Here's how the part is built. I have some questions about the finished solid (model axes, mm). Round coordinates to 2 decimals unless told otherwise and drop trailing zeros. Loops run counter-clockwise (first coordinate to the right, second up) from the corner with the lowest first, then second, coordinate; pieces in that order, holes last. Notation, with made-up numbers: (3.25, 41.25) - (37.25, 41.25) arc R29 cw to (37.25, 75.25) - close; hole circle Ø1 at (-29, -30.5). An arc over 180 degrees is marked (long way). Return JSON: item names as keys, results as strings. Group by question number.
```python
from build123d import *

# Parameters (mm, degrees)
SKETCH2_W                                     = 2006.6
SKETCH2_H                                     = 762
BOSS_EXTRUDE1_DEPTH                           = 25.4
BOSS_EXTRUDE4_DEPTH                           = 25.4
F_1_4_20_TAPPED_HOLE1_D                       = 5.1054
SKETCH5_R                                     = 215.9
CUT_EXTRUDE2_DEPTH                            = 26.4
SKETCH10_W                                    = 304.8
SKETCH10_H                                    = 762
CUT_EXTRUDE5_DEPTH                            = 26.4
SKETCH31_W                                    = 381
SKETCH31_H                                    = 82.55
CUT_EXTRUDE8_DEPTH                            = 26.4
CUT_EXTRUDE9_DEPTH                            = 26.4
CUT_EXTRUDE10_DEPTH                           = 26.4
SKETCH41_W                                    = 838.2
SKETCH41_H                                    = 457.2
CUT_EXTRUDE11_DEPTH                           = 26.4
CBORE_FOR_1_4_SOCKET_HEAD_CAP_SCREW1_AT_COUNT = 2
CBORE_FOR_1_4_SOCKET_HEAD_CAP_SCREW1_AT_PITCH = 204.781346807
CBORE_FOR_1_4_SOCKET_HEAD_CAP_SCREW1_2_COUNT  = 2
CBORE_FOR_1_4_SOCKET_HEAD_CAP_SCREW1_2_PITCH  = 618.530419624
CBORE_FOR_1_4_SOCKET_HEAD_CAP_SCREW1_3_COUNT  = 2
CBORE_FOR_1_4_SOCKET_HEAD_CAP_SCREW1_3_PITCH  = 819.912629492
CBORE_FOR_1_4_SOCKET_HEAD_CAP_SCREW1_4_COUNT  = 2
CBORE_FOR_1_4_SOCKET_HEAD_CAP_SCREW1_4_PITCH  = 813.196778154


with BuildPart() as part:
    # Sketch2 → Boss-Extrude1 (new body)
    with BuildSketch(Plane(origin=(0, 0, 0), x_dir=(1, 0, 0), z_dir=(0, 1, 0))):
        with Locations((596.720248579, 143.454782609)):
            Rectangle(SKETCH2_W, SKETCH2_H)
    extrude(amount=BOSS_EXTRUDE1_DEPTH)

    # Sketch63 → Boss-Extrude4 (add)
    with BuildSketch(Plane(origin=(0, 25.4, 0), x_dir=(1, 0, 0), z_dir=(0, 1, 0))):
        with BuildLine():
            Line((368.120248579, -237.545217391), (763.550813985, -237.545217391))
            Line((763.550813985, -237.545217391), (761.820248579, -275.645217391))
            Line((761.820248579, -275.645217391), (364.731895319, -275.645217391))
            ThreePointArc((364.731895319, -275.645217391), (367.271491927, -256.670403258), (368.120248579, -237.545217391))
        make_face()
    extrude(amount=-BOSS_EXTRUDE4_DEPTH)

    # 1/4-20 Tapped Hole1 (through all)
    with Locations(Plane(origin=(0, 25.4, 0), x_dir=(1, 0, 0), z_dir=(0, 1, 0))):
        with Locations((736.420248579, -262.945217391)):
            Hole(F_1_4_20_TAPPED_HOLE1_D / 2)

    # Sketch5 → Cut-Extrude2 (cut, through all)
    with BuildSketch(Plane(origin=(0, 25.4, 0), x_dir=(1, 0, 0), z_dir=(0, 1, 0))):
        with Locations((152.220248579, -237.545217391)):
            Circle(SKETCH5_R)
    extrude(amount=-CUT_EXTRUDE2_DEPTH, mode=Mode.SUBTRACT)

    # Sketch10 → Cut-Extrude5 (cut, through all)
    with BuildSketch(Plane(origin=(0, 25.4, 0), x_dir=(1, 0, 0), z_dir=(0, 1, 0))):
        with Locations((-254.179751421, 143.454782609)):
            Rectangle(SKETCH10_W, SKETCH10_H)
    extrude(amount=-CUT_EXTRUDE5_DEPTH, mode=Mode.SUBTRACT)

    # Sketch31 → Cut-Extrude8 (cut, through all)
    with BuildSketch(Plane(origin=(0, 25.4, 0), x_dir=(1, 0, 0), z_dir=(0, 1, 0))):
        with Locations((-216.079751421, -196.270217391)):
            Rectangle(SKETCH31_W, SKETCH31_H)
    extrude(amount=-CUT_EXTRUDE8_DEPTH, mode=Mode.SUBTRACT)

    # Sketch39 → Cut-Extrude9 (cut, through all)
    with BuildSketch(Plane(origin=(0, 25.4, 0), x_dir=(1, 0, 0), z_dir=(0, 1, 0))):
        with BuildLine():
            Line((-101.779751421, 480.875272294), (-101.779751421, 524.454782609))
            Line((-101.779751421, 524.454782609), (152.220248579, 524.454782609))
            ThreePointArc((152.220248579, 524.454782609), (23.36454079, 513.480885065), (-101.779751421, 480.875272294))
        make_face()
    extrude(amount=-CUT_EXTRUDE9_DEPTH, mode=Mode.SUBTRACT)

    # Sketch40 → Cut-Extrude10 (cut, through all)
    with BuildSketch(Plane(origin=(0, 25.4, 0), x_dir=(1, 0, 0), z_dir=(0, 1, 0))):
        with BuildLine():
            Line((152.220248579, 524.454782609), (1600.020248579, 524.454782609))
            Line((1600.020248579, 524.454782609), (1600.020248579, 219.654782609))
            Line((1600.020248579, 219.654782609), (761.820248579, 219.654782609))
            ThreePointArc((761.820248579, 219.654782609), (492.99700835, 444.008302151), (152.220248579, 524.454782609))
        make_face()
    extrude(amount=-CUT_EXTRUDE10_DEPTH, mode=Mode.SUBTRACT)

    # Sketch41 → Cut-Extrude11 (cut, through all)
    with BuildSketch(Plane(origin=(0, 25.4, 0), x_dir=(1, 0, 0), z_dir=(0, 1, 0))):
        with Locations((1180.920248579, -8.945217391)):
            Rectangle(SKETCH41_W, SKETCH41_H)
    extrude(amount=-CUT_EXTRUDE11_DEPTH, mode=Mode.SUBTRACT)

    # Sketch67 → CBORE for 1/4 Socket Head Cap Screw1 (revolve, cut)
    with BuildSketch(Plane(origin=(-76.379751421, 25.4, 8.945217391), x_dir=(0, 0, 1), z_dir=(1, 0, 0))):
        Polygon((0, 0), (0, 25.40005), (3.3782, 25.40005), (3.3782, 6.35), (5.55625, 6.35), (5.55625, 2.2225), (7.77875, 0), align=None)
    cbore_for_1_4_socket_head_cap_screw1 = revolve(axis=Axis((-76.379751421, 31.75, 8.945217391), (0, -1, 0)), mode=Mode.SUBTRACT)

    # CBORE for 1/4 Socket Head Cap Screw1 at: CBORE for 1/4 Socket Head Cap Screw1 ×2
    with Locations(*[Vector(0.124034735, 0, -0.992277877) * (i * CBORE_FOR_1_4_SOCKET_HEAD_CAP_SCREW1_AT_PITCH) for i in range(1, CBORE_FOR_1_4_SOCKET_HEAD_CAP_SCREW1_AT_COUNT)]):
        add(cbore_for_1_4_socket_head_cap_screw1, mode=Mode.SUBTRACT)

    # CBORE for 1_4 Socket Head Cap Screw1 2: CBORE for 1/4 Socket Head Cap Screw1 ×2
    with Locations(*[Vector(0.944496797, 0, -0.328520625) * (i * CBORE_FOR_1_4_SOCKET_HEAD_CAP_SCREW1_2_PITCH) for i in range(1, CBORE_FOR_1_4_SOCKET_HEAD_CAP_SCREW1_2_COUNT)]):
        add(cbore_for_1_4_socket_head_cap_screw1, mode=Mode.SUBTRACT)

    # CBORE for 1_4 Socket Head Cap Screw1 3: CBORE for 1/4 Socket Head Cap Screw1 ×2
    with Locations(*[Vector(0.960346227, 0, 0.278810195) * (i * CBORE_FOR_1_4_SOCKET_HEAD_CAP_SCREW1_3_PITCH) for i in range(1, CBORE_FOR_1_4_SOCKET_HEAD_CAP_SCREW1_3_COUNT)]):
        add(cbore_for_1_4_socket_head_cap_screw1, mode=Mode.SUBTRACT)

    # CBORE for 1_4 Socket Head Cap Screw1 4: CBORE for 1/4 Socket Head Cap Screw1 ×2
    with Locations(*[Vector(0.968277324, 0, -0.249878019) * (i * CBORE_FOR_1_4_SOCKET_HEAD_CAP_SCREW1_4_PITCH) for i in range(1, CBORE_FOR_1_4_SOCKET_HEAD_CAP_SCREW1_4_COUNT)]):
        add(cbore_for_1_4_socket_head_cap_screw1, mode=Mode.SUBTRACT)


solid = part.part
```
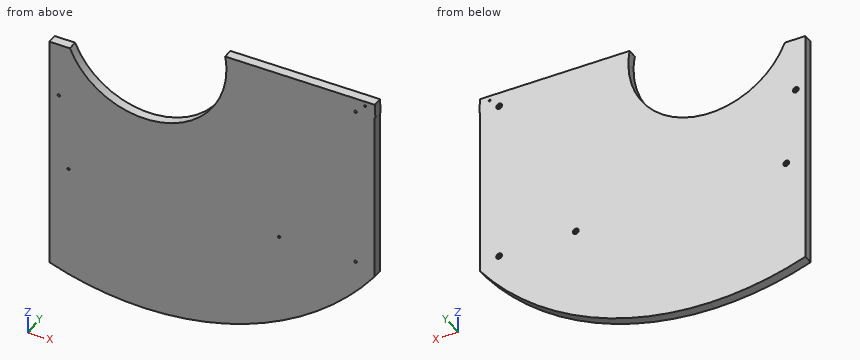
Q1. Imagine slicing it at B-B, the plane y = 6.25. List the corners of the cut face in (x, z) for me.
Q2. Will these pins go through, and if not, where does the flat tip stop? pin 1 Ø14.5 at (x, z) = (-50.98, -194.25) entering from +Y; pin 2 Ø0.9 at (x, y) = (762.5, 8) entering from -Z; pin 3 Ø10 at (x, y) = (267, 22) entering from +Z.
Q3. Imagine slicing it at A-A, the plane z = 99.5. List the corners of the cut face in (x, y) for me.
Q4. Imagine slicing it at C-C, the plane x = 118. List the corners of the cut face in (y, z) for me.
Q5. Imagine slicing it at D-D, the plane z = -395. List the corners of the cut face in (x, y) for me.
Q6. Please list where these lines run through material, in increasing order: line 1 (X direction, y = 11.75, z = -164); line 2 (X direction, y = 23.5, z = 10); line 3 (X direction, y = 5.75, z = 44).
Output values:
{
 "1": {"outline": "(-101.78, -480.88) arc R762 ccw to (761.82, -219.65) - (761.82, 237.55) - (763.55, 237.55) - (761.82, 275.65) - (364.73, 275.65) arc R215.9 cw to (-47.27, 155) - (-101.78, 155) - close; hole circle Ø6.76 at (-76.38, 8.95); hole circle Ø6.76 at (-50.98, -194.25); hole circle Ø6.76 at (507.82, -194.25); hole circle Ø6.76 at (711.02, -194.25); hole circle Ø6.76 at (711.02, 237.55); hole circle Ø5.11 at (736.42, 262.95)"},
 "2": {"pin 1": "stops at y = 24.88", "pin 2": "stops at z = 237.55", "pin 3": "stops at z = 57.92"},
 "3": {"outline": "(-101.78, 0) - (-13.78, 0) - (-13.78, 25.4) - (-101.78, 25.4) - close; (318.22, 0) - (761.82, 0) - (761.82, 25.4) - (318.22, 25.4) - close"},
 "4": {"outline": "(0, -523.69) - (25.4, -523.69) - (25.4, 24.37) - (0, 24.37) - close"},
 "5": {"outline": "(-101.78, 0) - (577.11, 0) - (577.11, 25.4) - (-101.78, 25.4) - close"},
 "6": {"line 1": "x = -101.78 to 761.82", "line 2": "x = -101.78 to -82.16, -70.6 to 761.82", "line 3": "x = -101.78 to 56.55, 247.89 to 761.82"}
}
